Design review of the part built by this model. Coordinates are the model's own, in mm. Face numbers are marked on the shaded views. A direction names the side the tool comes from. Give positions to 0.01 mm unless a question says otherwise; leave off trailing zeros. Order: outer loops, then holes, each group sorted by start corner. A loop starts at its lowest first (then second) coordinate and runs counter-clockwise, first axis right, second up. Notation, with made-up numbers: (-6, 34.25) -> (5, 34.25) arc R31 cw to (5, 61.25) -> close; hole circle Ø1 at (33.5, 15.25). An arc over 180 degrees is marked (long way). One line per item, written item: value.
from build123d import *

# Parameters (mm, degrees)
F0_R     = 4
F0_W     = 10
F0_H     = 25
F1_DEPTH = 15
F2_R     = 4.99999


# Not quite as in the source:
# - a fillet or chamfer is up to 0.001 mm smaller than in the source, because OpenCascade refuses the exact size


with BuildPart() as f1:
    # F0 (on Front) → F1 (new body)
    with BuildSketch(Plane.XZ):
        Polygon((56, 7.5), (-94, 7.5), (-94, -7.5), (-84, -7.5), (46, -7.5), (56, -7.5), align=None)
        with Locations((-84, 0)):
            Circle(F0_R, mode=Mode.SUBTRACT)
        Circle(F0_R, mode=Mode.SUBTRACT)
        with Locations((-89, -20)):
            Rectangle(F0_W, F0_H)
        with Locations((51, -20)):
            Rectangle(F0_W, F0_H)
    extrude(amount=F1_DEPTH)

    # F2 (radius 5 in the source; OpenCascade refuses exactly that, so slightly less here)
    f2_edges = [f1.edges().sort_by_distance(p)[0] for p in [
        (-84, -7.5, -7.5),
        (46, -7.5, -7.5),
        (56, -7.5, 7.5),
        (56, -7.5, -32.5),
        (46, -7.5, -32.5),
        (-94, -7.5, -32.5),
        (-84, -7.5, -32.5),
        (-94, -7.5, 7.5),
    ]]
    fillet(f2_edges, radius=F2_R)


solid = f1.part
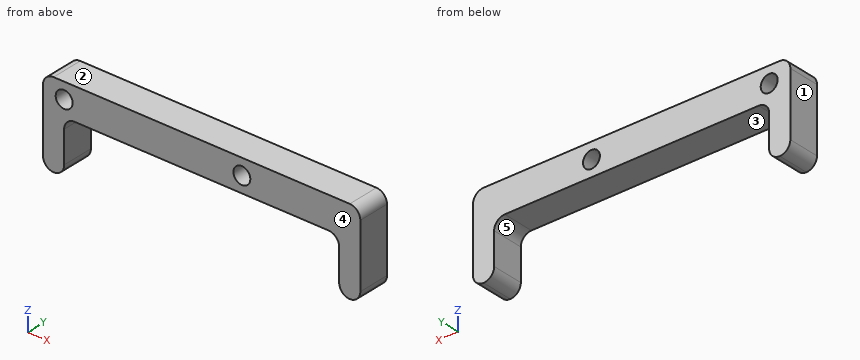
Item 1: Add section B-B on z = 0. Give the boundary of the cut face in (x, y).
Returned:
outline: (-94, -15) -> (-88, -15) -> (-88, 0) -> (-94, 0) -> close; (-80, -15) -> (-4, -15) -> (-4, 0) -> (-80, 0) -> close; (4, -15) -> (56, -15) -> (56, 0) -> (4, 0) -> close
Item 2: To check wall thickness, follow line 1 along X through (y, z) = (-9.75, -23.5); line 2 along X through (y, z) = (-6.5, -2.5); line 3 along Z through (x, y) = (0, -6.25). State the ranges of each line that lie inside material, in increasing order. Write a range as from..to.
Returned:
line 1: -94..-84, 46..56
line 2: -94..-87.12, -80.88..-3.12, 3.12..56
line 3: -7.5..-4, 4..7.5
Item 3: Add section D-D on z = -21. Give the boundary of the cut face in (x, y).
Returned:
outline: (-94, -15) -> (-84, -15) -> (-84, 0) -> (-94, 0) -> close; (46, -15) -> (56, -15) -> (56, 0) -> (46, 0) -> close
Item 4: Draft analysis for pull direction X (two halves, no side actions). For the marked faces 1, 2 and 3, state which applies: pulls with the +X half, pulls with the -X half, needs draft (parallel to the pull), parting line crosses it, or undercut.
Returned:
face 1: pulls with the -X half
face 2: needs draft
face 3: undercut
Item 5: Add section C-C on y = -3.25. Count the separate pieces of the cut face and the enclosed holes in it, plus the area to 3 significant figures.
Returned:
separate pieces: 1
enclosed holes: 2
area: 2,630 mm²
Item 6: Clearance check with a flat-ended pin moving along its axis: P1, Ø4, axis at x = 4.5, y = -10, coming from the -Z side. State where the tip first meets the part, or that it passes through.
Returned:
P1: z = -7.5
Item 7: Machinability: for the marked faces 4 and 5, which of the approach directions +Z, -Z, +X, -X, +Y, -Y give a long, thin tool a straight path to every point of the face, cutting with its end or side? Answer none if there is none.
Returned:
face 4: +Z, -Z, +X, -X, -Y
face 5: -Z, +Y, -Y
Item 8: Add section A-A on x = 0. Give the boundary of the cut face in (y, z), plus the area to 3 significant figures.
Returned:
outline: (-15, -7.5) -> (0, -7.5) -> (0, -4) -> (-15, -4) -> close; (-15, 4) -> (0, 4) -> (0, 7.5) -> (-15, 7.5) -> close
area: 105 mm²
